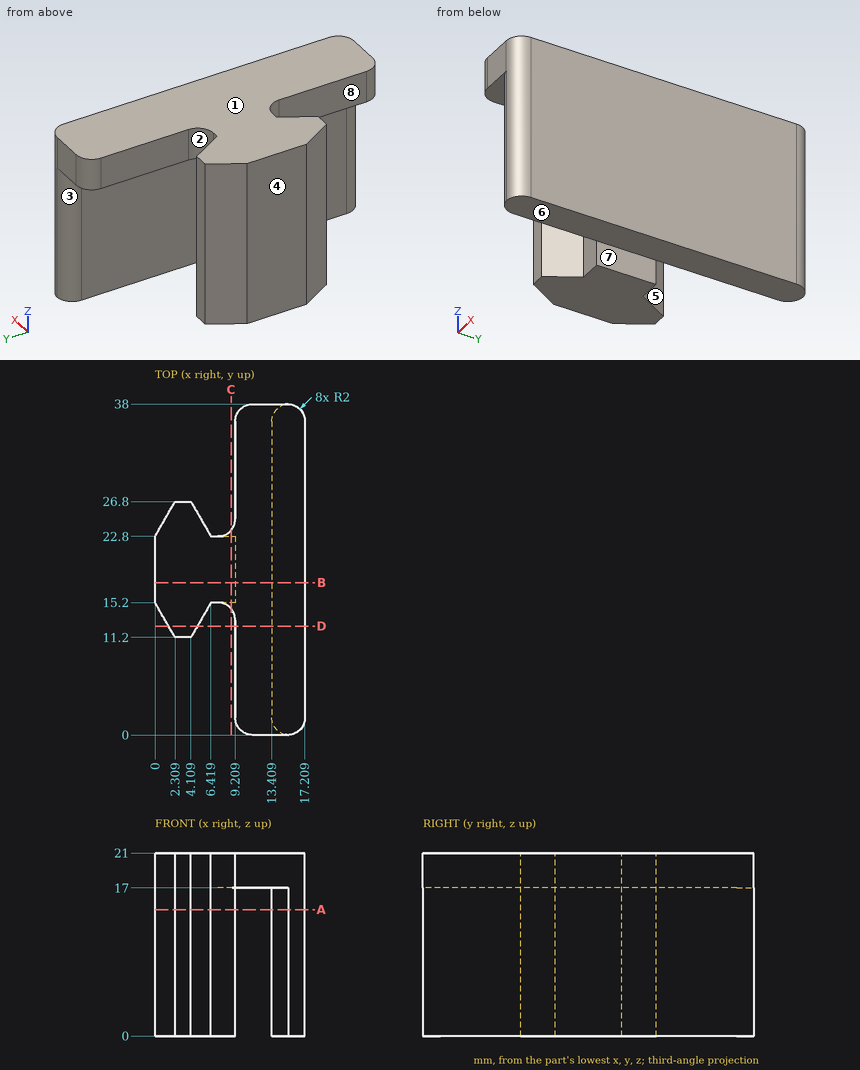
Print and shaded views of the part. All mm, measured from the part's lowest x, y and z. A direction names the side the tool comes from. Give positions to 0.01 mm unless a question says otherwise; leave off trailing zeros. Write each loop counter-clockwise with the first axis right and the second up, starting at its lowest first coordinate (ties: lowest second). Pieces come first, ordered by that corner, then holes. Notation, with made-up numbers: (18, 52) -> (48, 52) arc R17 cw to (48, 82) -> close; hole circle Ø7 at (43.5, 1). An arc over 180 degrees is marked (long way). Use CSV: the item, a comma, the result in double quotes. Start each with the question number.
1) Drill centre lines: L1, parallel to X at y = 15.5, z = 12.5; L2, parallel to X at y = 6.5, z = 2.5; L3, parallel to X at y = 23, z = 8 (1 decimal). Where is each one in solid material? Low to high.
2) Cut at D-D on y = 12.5. List the corners of the cut face in (x, z).
3) Cut at B-B on y = 17.5. List the corners of the cut face in (x, z).
4) Tool access for the marked faces 4, 5, 6, 7 and 8: list every direction of +Z, -Z, +X, -X, +Y, -Y with a clear straight run to the whole face (end or side of a thin tool).
5) Cut at C-C on x = 8.75. List the corners of the cut face in (y, z) (1 decimal).
6) Pin check, flat tips, straight feed: P1, Ø4.5, axis at y = 9.5, z = 20, coming from the -X side; P2, Ø2, axis at y = 32.5, z = 18, coming from the -X side; P3, Ø2, axis at x = 3.5, z = 7.5, coming from the +Y side. Stop position of each tip, or through.
7) Cut at A-A on z = 14.5. List the corners of the cut face in (x, y).
8) Two-plate mould, pull along X, no slides. Class the marked faces 1, 2 and 3: released by +X, released by -X, zero draft, split by the parting line, or undercut.
Final values:
1,L1,"x = 0 to 9.21, 13.41 to 17.21"
1,L2,"x = 13.41 to 17.21"
1,L3,"x = 0.1 to 6.3, 13.4 to 17.2"
2,outline,"(1.56, 0) -> (4.86, 0) -> (4.86, 21) -> (1.56, 21) -> close; (9.21, 17) -> (13.41, 17) -> (13.41, 0) -> (17.21, 0) -> (17.21, 21) -> (9.21, 21) -> close"
3,outline,"(0, 0) -> (9.21, 0) -> (9.21, 17) -> (13.41, 17) -> (13.41, 0) -> (17.21, 0) -> (17.21, 21) -> (0, 21) -> close"
4,face 4,"+Z, -Z, -X, +Y, -Y"
4,face 5,"+Z, -Z, +Y"
4,face 6,"-Z, +X, -X, +Y, -Y"
4,face 7,"-Z, +Y, -Y"
4,face 8,"+Z, -Z, -Y"
5,outline,"(14.5, 17) -> (15.2, 17) -> (15.2, 0) -> (22.8, 0) -> (22.8, 17) -> (23.5, 17) -> (23.5, 21) -> (14.5, 21) -> close"
6,P1,"stops at x = 1.99"
6,P2,"stops at x = 9.21"
6,P3,"stops at y = 26.8"
7,outline,"(0, 15.2) -> (2.31, 11.2) -> (4.11, 11.2) -> (6.42, 15.2) -> (9.21, 15.2) -> (9.21, 22.8) -> (6.42, 22.8) -> (4.11, 26.8) -> (2.31, 26.8) -> (0, 22.8) -> close; (13.41, 2) arc R2 ccw to (15.31, 0) arc R2 ccw to (17.21, 2) -> (17.21, 36) arc R2 ccw to (15.31, 38) arc R2 ccw to (13.41, 36) -> close"
8,face 1,"zero draft"
8,face 2,"undercut"
8,face 3,"released by -X"
